The listing builds one solid part. Answer for the finished solid, in the listing's coordinates (mm). Face numbers are marked on the shaded views. A direction names the side the tool comes from. Coordinates: 2 decimals unless noted, no trailing zeros. Write each loop counter-clockwise with the first axis right and the second up, starting at its lowest first coordinate (ties: lowest second). Pieces come first, ordered by that corner, then holes.
from build123d import *

# Parameters (mm, degrees)
F0_R     = 31.75
F1_DEPTH = 12.7
F2_R     = 15.875
F3_DEPTH = 12.7
F4_R     = 3.175
F5_DEPTH = 12.701


with BuildPart() as f1:
    # F0 (on Top) → F1 (new body)
    with BuildSketch(Plane.XY):
        Circle(F0_R)
    extrude(amount=F1_DEPTH)

    # F2 (on face) → F3 (join)
    with BuildSketch(Plane.XY.offset(12.7)):
        Circle(F2_R)
    extrude(amount=F3_DEPTH)

    # F4 (on face) → F5 (cut, through all)
    with BuildSketch(Plane.XY.offset(12.7)):
        with Locations((25.4, 0)):
            Circle(F4_R)
        with Locations((0, 25.4)):
            Circle(F4_R)
        with Locations((-25.4, 0)):
            Circle(F4_R)
        with Locations((0, -25.4)):
            Circle(F4_R)
    extrude(amount=-F5_DEPTH, mode=Mode.SUBTRACT)


solid = f1.part
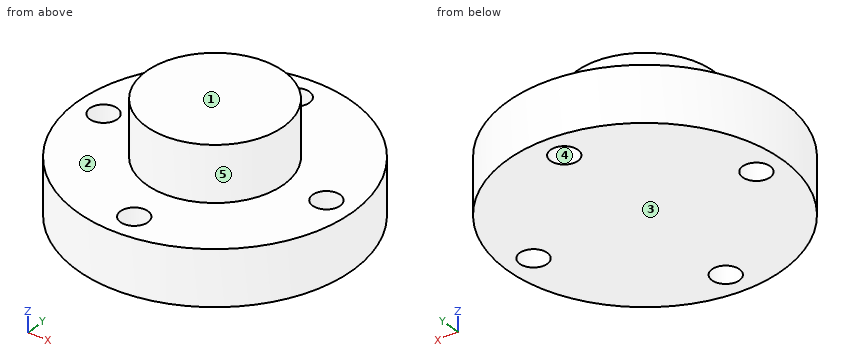
Q1. Find the intervals of material crossed by probe 1 along Y at (x, z) = (0, 10.25) (3 decimals); probe 2 along Z at (x, y) = (-11, 23); probe 3 along X at (y, z) = (-1, 11), in increasing order.
Answers below:
probe 1: y = -31.75 to -28.575, -22.225 to 22.225, 28.575 to 31.75
probe 2: z = 0 to 12.7
probe 3: x = -31.73 to -28.41, -22.39 to 22.39, 28.41 to 31.73
Q2. Determine the mould class of the marked faces 3, 4 and 5 for opening direction Y: released by +Y, released by -Y, zero draft, split by the parting line, or undercut.
Answers below:
face 3: zero draft
face 4: undercut
face 5: split by the parting line
Q3. The part is cut by section A-A, the plane x = 0. Write down the section's boundary in (y, z) (3 decimals), then the cut area to 3 significant figures.
Answers below:
outline: (-31.75, 0) - (-28.575, 0) - (-28.575, 12.7) - (-31.75, 12.7) - close; (-22.225, 0) - (22.225, 0) - (22.225, 12.7) - (15.875, 12.7) - (15.875, 25.4) - (-15.875, 25.4) - (-15.875, 12.7) - (-22.225, 12.7) - close; (28.575, 0) - (31.75, 0) - (31.75, 12.7) - (28.575, 12.7) - close
area: 1,050 mm2
Q4. Given pin 1 (6 mm diameter, centred on x = 1.5, y = -19, fed in from +Z); pin 2 (3 mm diameter, centred on x = -10, y = 3.5, fed in from -Z); pin 3 (12 mm diameter, centred on y = -8.5, z = 11, fed in from -X); pin 4 (2 mm diameter, centred on x = -14.5, z = 16, fed in from -Y), each flat-ended and moving along its own axis, determine where each tip first touches the part or whether it passes through.
Answers below:
pin 1: stops at z = 12.7
pin 2: stops at z = 0
pin 3: stops at x = -31.65
pin 4: stops at y = -8.35
Q5. The part is cut by section C-C, the plane x = 25.4. Write down the section's boundary in (y, z) (3 decimals).
Answers below:
outline: (-19.05, 0) - (-3.175, 0) - (-3.175, 12.7) - (-19.05, 12.7) - close; (3.175, 0) - (19.05, 0) - (19.05, 12.7) - (3.175, 12.7) - close
Q6. Which of the six approach directions +Z, -Z, +X, -X, +Y, -Y give full straight-line access (tool end or side, diameter ignored) to the marked faces 1 and 2?
Answers below:
face 1: +Z, +X, -X, +Y, -Y
face 2: +Z
